Check sheet for the modelled part. Datum: model origin and axes. Units: mm. Face numbers are marked on the shaded views. A direction names the side the tool comes from. Coordinates: 2 decimals unless noted, no trailing zeros. Loops run counter-clockwise (first coordinate to the right, second up) from the corner with the lowest first, then second, coordinate; pieces in that order, holes last. Notation, with made-up numbers: (18.5, 21.25) - (51.5, 21.25) arc R33 cw to (51.5, 56.25) - close; hole circle Ø4 at (40.25, -1). An arc over 180 degrees is marked (long way). Use a Markdown table: item, result. Add a question column.
1) Draft check along X on the marked faces 5, 6 and 7. Enter one of: pulls with the +X half, pulls with the -X half, needs draft (parallel to the pull), parting line crosses it, or undercut.
2) Sectioned sample at B-B, the plane y = 1.25. Enter the section's corners in (x, z).
3) Thickness scan on line 1 (Y direction, x = 0, z = 1.85); line 2 (Y direction, x = 60.96, z = 1.7); line 3 (X direction, y = -7.5, z = 23.75). Record the ranges inside material, lowest first.
4) Sectioned sample at A-A, the plane x = 0. Enter the section's corners in (y, z), then the cut area to 3 significant figures.
5) Tool access check on the marked faces 1, 2, 3 and 4. Record the directions out of +Z, -Z, +X, -X, +Y, -Y that give a thin tool (end or side, any length) a straight path to the whole face; none if there is none.
6) Sectioned sample at D-D, the plane x = 60.96. Enter the section's corners in (y, z), then the cut area to 3 significant figures.
7) Go/stop test with flat-tipped pins: P1, Ø2.5, axis at y = -1, z = 12.5, coming from the +X side; P2, Ø4, axis at x = 18, y = -2.5, coming from the +Z side; P3, Ø3, axis at x = 59.5, z = 10.5, coming from the +Y side; P4, Ø1.5, axis at x = 49.5, y = -1, coming from the +Z side. Record where each tip stops, or that it passes through.
8) Sectioned sample at C-C, the plane z = 23.75. Enter the section's corners in (x, y).
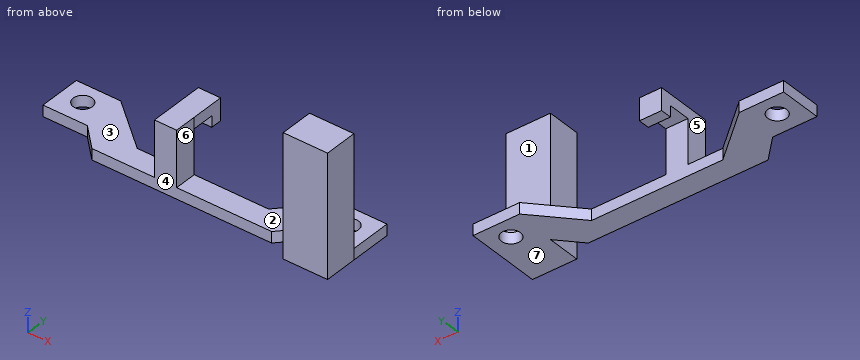
from build123d import *

# Parameters (mm, degrees)
SKETCH1_R                = 2.1717
BOSS_EXTRUDE2_DEPTH      = 2.54
BOSS_EXTRUDE3_DEPTH      = 25.4
BOSS_EXTRUDE3_DEPTH_BACK = 2.54
SKETCH3_W                = 5.074384234
SKETCH3_H                = 5.076844133
BOSS_EXTRUDE4_DEPTH      = 12.7
BOSS_EXTRUDE5_DEPTH      = 5.08


with BuildPart() as part:
    # Sketch1 → Boss-Extrude2 (new body)
    with BuildSketch(Plane.XY):
        Polygon((5.08, -5.08), (-5.08, -5.08), (-5.08, 4.572), (5.08, 4.572), (16.444283816, -5.025270266), (46.498564563, -5.025270266), (55.358360552, 4.543956213), (66.03999997, 4.543956213), (66.03999997, -5.052635133), (55.90534362, -5.052635133), (51.228827675, -10.102114399), (10.102114399, -10.102114399), align=None)
        Circle(SKETCH1_R, mode=Mode.SUBTRACT)
        with Locations((60.96, 0)):
            Circle(SKETCH1_R, mode=Mode.SUBTRACT)
    extrude(amount=BOSS_EXTRUDE2_DEPTH)

    # Sketch2 → Boss-Extrude3 (add, two sides: drawn at the far end of the back side and taken through both)
    with BuildSketch(Plane.XY.offset(2.54).offset(-BOSS_EXTRUDE3_DEPTH_BACK)):
        Polygon((55.90534362, -5.052635133), (55.90534362, -12.672635133), (66.06534362, -12.672635133), (66.03999997, -5.052635133), align=None)
    extrude(amount=BOSS_EXTRUDE3_DEPTH + BOSS_EXTRUDE3_DEPTH_BACK)

    # Sketch3 → Boss-Extrude4 (add)
    with BuildSketch(Plane.XY.offset(2.54)):
        with Locations((26.948840143, -7.563692333)):
            Rectangle(SKETCH3_W, SKETCH3_H)
    extrude(amount=BOSS_EXTRUDE4_DEPTH)

    # Sketch5 → Boss-Extrude5 (add)
    with BuildSketch(Plane.ZY.offset(-24.411648026)):
        Polygon((15.24, -5.025270266), (15.24, 2.594729734), (12.699847587, 2.594729734), (10.159847587, 2.594729734), (10.159847587, 0.054729734), (12.699847587, 0.054729734), (12.699847587, -5.025270266), align=None)
    extrude(amount=-BOSS_EXTRUDE5_DEPTH)


solid = part.part
Solved:
| question | item | result |
|---|---|---|
| 1 | face 5 | pulls with the -X half |
| 1 | face 6 | undercut |
| 1 | face 7 | needs draft |
| 2 | outline | (-5.08, 0) - (-1.78, 0) - (-1.78, 2.54) - (-5.08, 2.54) - close; (1.78, 0) - (9.01, 0) - (9.01, 2.54) - (1.78, 2.54) - close; (24.41, 10.16) - (29.49, 10.16) - (29.49, 15.24) - (24.41, 15.24) - close; (52.31, 0) - (59.18, 0) - (59.18, 2.54) - (52.31, 2.54) - close; (62.74, 0) - (66.04, 0) - (66.04, 2.54) - (62.74, 2.54) - close |
| 3 | line 1 | y = -5.08 to -2.17, 2.17 to 4.57 |
| 3 | line 2 | y = -12.67 to -2.17, 2.17 to 4.54 |
| 3 | line 3 | x = 55.91 to 66.05 |
| 4 | outline | (-5.08, 0) - (-2.17, 0) - (-2.17, 2.54) - (-5.08, 2.54) - close; (2.17, 0) - (4.57, 0) - (4.57, 2.54) - (2.17, 2.54) - close |
| 4 | area | 13.5 mm2 |
| 5 | face 1 | +Z, +X, +Y |
| 5 | face 2 | +Z, +Y |
| 5 | face 3 | +Z, -X, +Y, -Y |
| 5 | face 4 | +Z, -Z, -X, -Y |
| 6 | outline | (-12.67, 0) - (-2.17, 0) - (-2.17, 2.54) - (-5.05, 2.54) - (-5.05, 27.94) - (-12.67, 27.94) - close; (2.17, 0) - (4.54, 0) - (4.54, 2.54) - (2.17, 2.54) - close |
| 6 | area | 226 mm2 |
| 7 | P1 | stops at x = 29.49 |
| 7 | P2 | passes through |
| 7 | P3 | stops at y = -5.05 |
| 7 | P4 | stops at z = 2.54 |
| 8 | outline | (55.91, -12.67) - (66.07, -12.67) - (66.04, -5.05) - (55.91, -5.05) - close |
